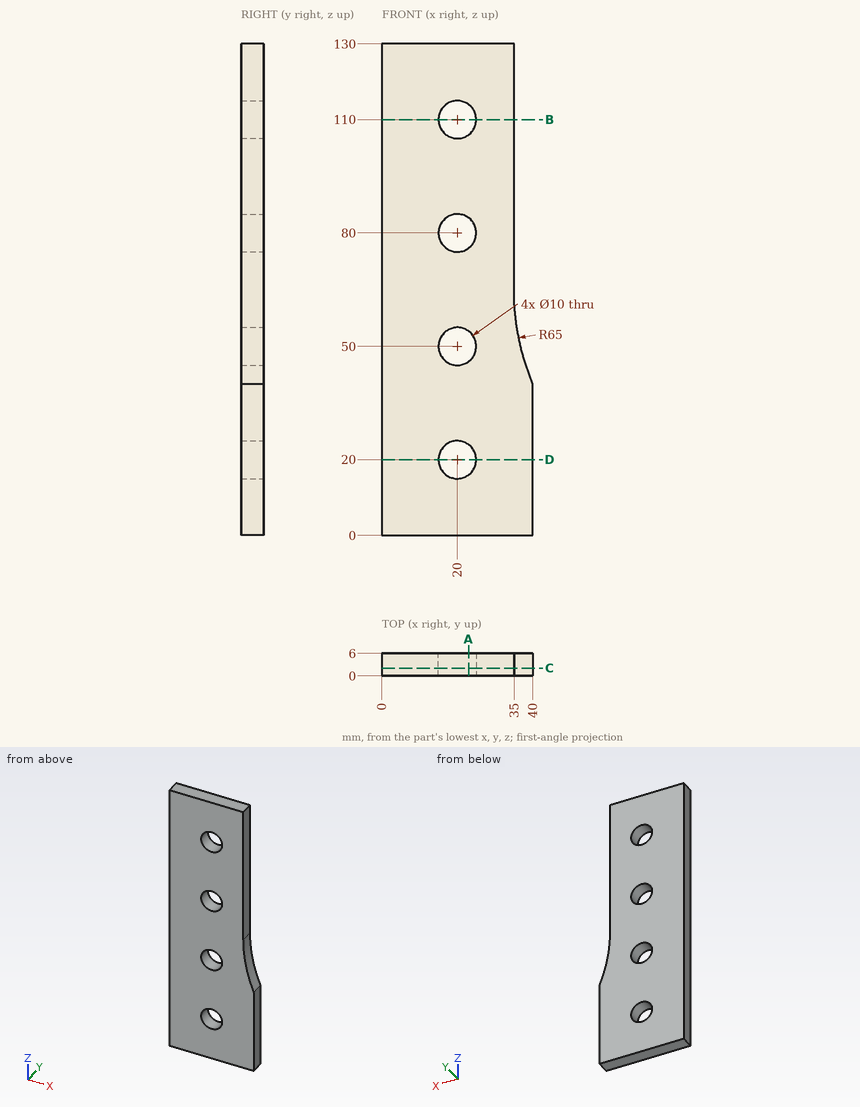
The figure shows three views and two pictorial views of one solid part (mm, origin at its lowest corner). Answer the questions. Coordinates: 2 decimals unless noted, no trailing zeros. Write each loop counter-clockwise with the first axis right and the second up, starting at its lowest first coordinate (ties: lowest second). Pieces come first, ordered by that corner, then holes. Notation, with made-up numbers: (83, -7.5) -> (123, -7.5) arc R17 ccw to (123, 5.5) -> close; hole circle Ø1 at (75, -38). An arc over 180 degrees is marked (long way). Answer as a JSON object with one key per item and string values.
Q1. The part is cut by section D-D on z = 20. Give the vertices of the cut face in (x, y), then the cut area to 3 significant figures.
The answers:
{"outline": "(0, 0) -> (15, 0) -> (15, 6) -> (0, 6) -> close; (25, 0) -> (40, 0) -> (40, 6) -> (25, 6) -> close", "area": "180 mm2"}
Q2. The part is cut by section B-B on z = 110. Give the vertices of the cut face in (x, y).
The answers:
{"outline": "(0, 0) -> (15, 0) -> (15, 6) -> (0, 6) -> close; (25, 0) -> (35, 0) -> (35, 6) -> (25, 6) -> close"}
Q3. The part is cut by section C-C on y = 2.1. Give the vertices of the cut face in (x, z).
The answers:
{"outline": "(0, 0) -> (40, 0) -> (40, 40) arc R65 cw to (35, 65) -> (35, 130) -> (0, 130) -> close; hole circle Ø10 at (20, 20); hole circle Ø10 at (20, 50); hole circle Ø10 at (20, 80); hole circle Ø10 at (20, 110)"}
Q4. The part is cut by section A-A on x = 23. Give the vertices of the cut face in (y, z), then the cut area to 3 significant figures.
The answers:
{"outline": "(0, 0) -> (6, 0) -> (6, 16) -> (0, 16) -> close; (0, 24) -> (6, 24) -> (6, 46) -> (0, 46) -> close; (0, 54) -> (6, 54) -> (6, 76) -> (0, 76) -> close; (0, 84) -> (6, 84) -> (6, 106) -> (0, 106) -> close; (0, 114) -> (6, 114) -> (6, 130) -> (0, 130) -> close", "area": "588 mm2"}
Q5. A flat-ended cylindrical pin translates along its axis: pin 1 Ø6 at (x, z) = (20, 80) entering from -Y. Find the tip coordinate at first contact, or state that the pin passes through.
The answers:
{"pin 1": "passes through"}
Q6. Consider line 1 (Z direction, x = 20, y = 4.7); line 2 (Z direction, x = 22, y = 1.45); line 3 (X direction, y = 3.2, z = 20.5). Determine where each line is inside the solid, lowest interval first. Write a range as [from, to].
The answers:
{"line 1": "z = [0, 15], [25, 45], [55, 75], [85, 105], [115, 130]", "line 2": "z = [0, 15.42], [24.58, 45.42], [54.58, 75.42], [84.58, 105.42], [114.58, 130]", "line 3": "x = [0, 15.03], [24.97, 40]"}
